Autodesk Inventor part; units mm, degrees
ref_plane "YZ Plane" through (0, 0, 0) normal (1, 0, 0) x (0, 1, 0)
ref_plane "XZ Plane" through (0, 0, 0) normal (0, 1, 0) x (-1, 0, 0)
ref_plane "XY Plane" through (0, 0, 0) normal (0, 0, 1) x (1, 0, 0)
sketch "スケッチ1" plane through (0, 0, 0) normal (0, 0, 1) x (1, 0, 0)
  circle A0 centre (0, 0) radius 4
  circle A1 centre (0, 0) radius 2
  dimension "d0" = 8
  dimension "d1" = 4
extrude "押し出し1" add sketch "スケッチ1" along normal blind 38 contours A0 | A1
sketch "スケッチ2" plane through (0, 0, 38) normal (0, 0, 1) x (1, 0, 0)
  circle A0 centre (0, 0) radius 1.5
  dimension "d4" = 3
extrude "押し出し2" cut sketch "スケッチ2" against normal blind 8
sketch "スケッチ3" plane through (0, 0, 0) normal (0, 0, -1) x (-1, 0, 0)
  circle A0 centre (0, 0) radius 1.5
  dimension "d7" = 3
extrude "押し出し3" cut sketch "スケッチ3" against normal blind 8
properties part number "スペーサーm3,38,Φ8,自作" material "アルミニウム 7075"
Model file for the job. Use its own axes, mm. A direction names the side the tool comes from. Give positions to 0.01 mm unless a question says otherwise; leave off trailing zeros. Order: outer loops, then holes, each group sorted by start corner. A loop starts at its lowest first (then second) coordinate and runs counter-clockwise, first axis right, second up. Notation, with made-up numbers: (44.5, 69) - (60.5, 69) arc R11 cw to (60.5, 81) - close; hole circle Ø9 at (41, 82.5). An arc over 180 degrees is marked (long way). One line per item, written item: value.
Item 1: Two-plate mould, pull along Y, no slides. Class faces 1 (the flat face through (0, 0, 8)), 2 (the flat face through (2, 0, 38)), 3 (the cylindrical face through (-0.867, 3.905, 18.734)), 4 (the cylindrical face through (1.5, 0.07, 3.94)): released by +Y, released by -Y, zero draft, split by the parting line, or undercut.
Response values:
face 1: undercut
face 2: zero draft
face 3: split by the parting line
face 4: undercut
Item 2: Slice it at A-A (y = 0). List the corners of the cut face in (x, z).
Response values:
outline: (-4, 0) - (-1.5, 0) - (-1.5, 8) - (1.5, 8) - (1.5, 0) - (4, 0) - (4, 38) - (1.5, 38) - (1.5, 30) - (-1.5, 30) - (-1.5, 38) - (-4, 38) - close
Item 3: Tool access for faces 5 (the flat face through (0, 0, 30)), 6 (the flat face through (2, 0, 0)): list every direction of +Z, -Z, +X, -X, +Y, -Y with a clear straight run to the whole face (end or side of a thin tool).
Response values:
face 5: +Z
face 6: -Z, +X, -X, +Y, -Y
Item 4: Slice it at D-D (z = 22). List the corners of the cut face in (x, y).
Response values:
outline: circle Ø8 at (0, 0)
Item 5: Slice it at C-C (z = 33.5). List the corners of the cut face in (x, y), then the cut area to 3 significant figures.
Response values:
outline: circle Ø8 at (0, 0); hole circle Ø3 at (0, 0)
area: 43.2 mm2
Item 6: Pin check, flat tips, straight feed: pin 1 Ø2.5 at (x, y) = (0, 0) entering from -Z; pin 2 Ø1 at (x, z) = (-2, 12.5) entering from -Y; pin 3 Ø1.8 at (x, y) = (0, 0) entering from +Z. Stop position of each tip, or through.
Response values:
pin 1: z = 8
pin 2: y = -3.71
pin 3: z = 30
Item 7: Wall check: line 1 (Y direction, x = 0, z = 34.75); line 2 (X direction, y = 0.25, z = 23); line 3 (X direction, y = 0.75, z = 2.5). Give the ranges that are in metal, low to high.
Response values:
line 1: -4 to -1.5, 1.5 to 4
line 2: -3.99 to 3.99
line 3: -3.93 to -1.3, 1.3 to 3.93
